```python
from build123d import *

# Parameters (mm, degrees)
SKETCH4_R           = 2.5
BOSS_EXTRUDE1_DEPTH = 64.27
SKETCH5_R           = 2.5
CUT_EXTRUDE1_DEPTH  = 72.548291037
SKETCH6_R           = 2.5
CUT_EXTRUDE2_DEPTH  = 74.179063133
SKETCH7_R           = 3.25
CUT_EXTRUDE3_DEPTH  = 1
SKETCH8_R           = 3.25
CUT_EXTRUDE4_DEPTH  = 1


with BuildPart() as part:
    # Sketch4 → Boss-Extrude1 (new body)
    with BuildSketch(Plane(origin=(0, 0, 0), x_dir=(1, 0, 0), z_dir=(0, 1, 0))):
        with BuildLine():
            Line((-5.286754077, 14.301163994), (13.559651759, 14.301163994))
            Line((13.559651759, 14.301163994), (13.559651759, 19.301163994))
            Line((13.559651759, 19.301163994), (-6.440348241, 19.301163994))
            Line((-6.440348241, 19.301163994), (-6.440348241, 22.501163994))
            ThreePointArc((-6.440348241, 22.501163994), (-13.511416053, 19.572231806), (-16.440348241, 12.501163994))
            Line((-16.440348241, 12.501163994), (-13.240348241, 12.501163994))
            Line((-13.240348241, 12.501163994), (-13.240348241, -7.498836006))
            Line((-13.240348241, -7.498836006), (-8.240348241, -7.498836006))
            Line((-8.240348241, -7.498836006), (-8.240348241, 11.347569829))
            ThreePointArc((-8.240348241, 11.347569829), (-6.440348241, 12.501163994), (-5.286754077, 14.301163994))
        make_face()
        with Locations(Location((-9.975882147, 16.0366979, 0), (0, 0, 270))):
            Circle(SKETCH4_R, mode=Mode.SUBTRACT)
    extrude(amount=BOSS_EXTRUDE1_DEPTH)

    # Sketch5 → Cut-Extrude1 (cut, through all)
    with BuildSketch(Plane(origin=(0, 0, -19.301163994), x_dir=(-1, 0, 0), z_dir=(0, 0, -1))):
        with Locations((-3.559651759, 48.2025)):
            Circle(SKETCH5_R)
        with Locations((-3.559651759, 16.0675)):
            Circle(SKETCH5_R)
    extrude(amount=-CUT_EXTRUDE1_DEPTH, mode=Mode.SUBTRACT)

    # Sketch6 → Cut-Extrude2 (cut, through all)
    with BuildSketch(Plane.ZY.offset(13.240348241)):
        with Locations((-2.501163994, 48.2025)):
            Circle(SKETCH6_R)
        with Locations((-2.501163994, 16.0675)):
            Circle(SKETCH6_R)
    extrude(amount=-CUT_EXTRUDE2_DEPTH, mode=Mode.SUBTRACT)

    # Sketch7 → Cut-Extrude3 (cut)
    with BuildSketch(Plane(origin=(-8.240348241, 0, 0), x_dir=(0, 0, -1), z_dir=(1, 0, 0))):
        with Locations((2.501163994, 48.2025)):
            Circle(SKETCH7_R)
        with Locations((2.501163994, 16.0675)):
            Circle(SKETCH7_R)
    extrude(amount=-CUT_EXTRUDE3_DEPTH, mode=Mode.SUBTRACT)

    # Sketch8 → Cut-Extrude4 (cut)
    with BuildSketch(Plane.XY.offset(-14.301163994)):
        with Locations((3.559651759, 48.2025)):
            Circle(SKETCH8_R)
        with Locations((3.559651759, 16.0675)):
            Circle(SKETCH8_R)
    extrude(amount=-CUT_EXTRUDE4_DEPTH, mode=Mode.SUBTRACT)


solid = part.part
```
The model under review builds one solid part; all positions refer to its coordinate system, in mm. A direction names the side the tool comes from. Give positions to 0.01 mm unless a question says otherwise; leave off trailing zeros. Loops run counter-clockwise (first coordinate to the right, second up) from the corner with the lowest first, then second, coordinate; pieces in that order, holes last. Notation, with made-up numbers: (38.25, 62) - (68.25, 62) arc R35 cw to (68.25, 96) - close; hole circle Ø4 at (-18.5, 7.25). An arc over 180 degrees is marked (long way). Answer as a JSON object with one key per item and string values.
Q1. For faces 5 (the flat face through (4, 32, -19.301)), 6 (the flat face through (-13.24, 32, -3)), 7 (the cylindrical face through (2.855, 12.895, -14.794)), 8 (the flat face through (4, 32, -14.301)), list the 3-axis set-ups (+Z, -Z, +X, -X, +Y, -Y) from which the entire face can be reached by the end or side of a thin tool; tool diameter is ignored.
Worked out:
{"face 5": "-Z, +X, +Y, -Y", "face 6": "+Z, -X, +Y, -Y", "face 7": "+Z", "face 8": "+Z, +X, +Y, -Y"}
Q2. To check wall thickness, follow line 1 along Z through (x, y) = (-10.25, 50.5); line 2 along X through (y, z) = (60, 1); line 3 along Z through (x, y) = (7, 54). State the ranges of each line that lie inside material, in increasing order.
Worked out:
{"line 1": "z = -21.75 to -18.52, -13.55 to -3.49, -1.52 to 7.5", "line 2": "x = -13.24 to -8.24", "line 3": "z = -19.3 to -14.3"}
Q3. Mouldability with a two-part tool opening along Z and no side actions: class faces 1 (the cylindrical face through (3.137, 51.425, -14.794)), 2 (the flat face through (-9.24, 46, -4)), 3 (the flat face through (-15, 32, -12.501)), 4 (the cylindrical face through (-8.733, 12.895, -1.797)) as +Z half, -Z half, draft (parallel to the pull), parting line (faces both ways), or undercut.
Worked out:
{"face 1": "draft", "face 2": "undercut", "face 3": "+Z half", "face 4": "undercut"}
Q4. Insertion check: pin 1 (6 mm diameter, centred on x = 3.56, y = 48.2, fed in from -Z); pin 2 (3 mm diameter, centred on x = 9, y = 49, fed in from +Z); pin 3 (5 mm diameter, centred on x = 3, y = 48, fed in from +Z); pin 4 (10 mm diameter, centred on x = -2, z = -4.5, fed in from -Y). Each pin has a flat end and moves straight along its axis. Give the tip position at first contact, or say it passes through.
Worked out:
{"pin 1": "stops at z = -19.3", "pin 2": "stops at z = -14.3", "pin 3": "stops at z = -15.3", "pin 4": "passes through"}
Q5. Add section C-C on z = 4.5. State the section outline as (x, y) points.
Worked out:
{"outline": "(-13.24, 0) - (-8.24, 0) - (-8.24, 64.27) - (-13.24, 64.27) - close"}
Q6. Add section D-D on x = -3. State the section outline as (y, z) points, plus the area to 3 significant figures.
Worked out:
{"outline": "(0, -19.3) - (64.27, -19.3) - (64.27, -14.3) - (0, -14.3) - close", "area": "321 mm^2"}
Q7. Add section B-B on y = 11.5. State the section outline as (x, z) points.
Worked out:
{"outline": "(-16.44, -12.5) arc R10 ccw to (-6.44, -22.5) - (-6.44, -19.3) - (13.56, -19.3) - (13.56, -14.3) - (-5.29, -14.3) arc R5 ccw to (-8.24, -11.35) - (-8.24, 7.5) - (-13.24, 7.5) - (-13.24, -12.5) - close; hole circle Ø5 at (-9.98, -16.04)"}
Q8. Add section A-A on y = 49. State the section outline as (x, z) points, plus the area to 3 significant figures.
Worked out:
{"outline": "(-16.44, -12.5) arc R10 ccw to (-6.44, -22.5) - (-6.44, -19.3) - (1.19, -19.3) - (1.19, -15.3) - (0.41, -15.3) - (0.41, -14.3) - (-5.29, -14.3) arc R5 ccw to (-8.24, -11.35) - (-8.24, -5.65) - (-9.24, -5.65) - (-9.24, -4.87) - (-13.24, -4.87) - (-13.24, -12.5) - close; (-13.24, -0.13) - (-9.24, -0.13) - (-9.24, 0.65) - (-8.24, 0.65) - (-8.24, 7.5) - (-13.24, 7.5) - close; (5.93, -19.3) - (13.56, -19.3) - (13.56, -14.3) - (6.71, -14.3) - (6.71, -15.3) - (5.93, -15.3) - close; hole circle Ø5 at (-9.98, -16.04)", "area": "211 mm^2"}
